Print and shaded views of the part. All mm, measured from the part's lowest x, y and z. A direction names the side the tool comes from. Round coordinates to 2 decimals unless told otherwise and drop trailing zeros. Order: outer loops, then holes, each group sorted by start corner. A loop starts at its lowest first (then second) coordinate and runs counter-clockwise, first axis right, second up. Notation, with made-up numbers: (64, -10) - (85, -10) arc R22 ccw to (85, 28) - close; hole circle Ø9 at (33, 2.5). An arc over 180 degrees is marked (long way). Write item = value, one per line. Start each with the question number.
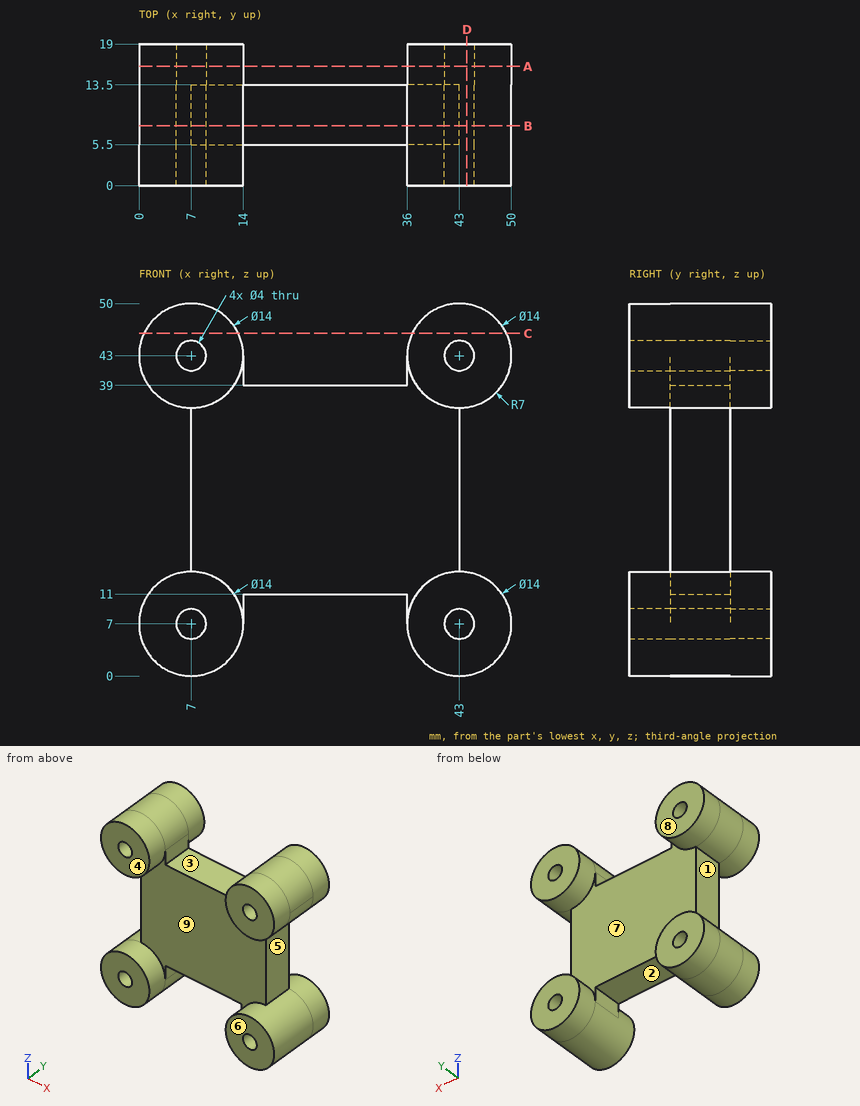
Item 1: Saw through at C-C, the plane z = 46. Give the cut face in (x, y), then the cut area to 3 significant figures.
Item 2: Mould opens along X. For the marked faces 1, 2, 3 and 4 say: +X half, -X half, draft (parallel to the pull), parting line (faces both ways), or undercut.
Item 3: Saw through at B-B, the plane y = 8. Give the cut face in (x, z).
Item 4: Probe L1, parallel to X at y = 17.35, z = 7; L2, parallel to Z at x = 32.5, y = 12.5. List the from-to ranges inside material, lowest first.
Item 5: Saw through at D-D, the plane x = 44. Give the cut face in (y, z).
Item 6: Which spindle directions (+Z, -Z, +X, -X, +Y, -Y) get a long thin tool onto all of the face, cutting with end or side? Do the marked faces 5, 6, 7, 8 and 9. Say none if no direction does.
Item 7: Saw through at A-A, the plane y = 16. Give the cut face in (x, z).
Item 8: Drop flat-ended pins along their axis: pin 1 (6 mm diameter, centred on x = 12.5, y = 4, fed in from +Z); pin 2 (1.2 mm diameter, centred on y = 11.5, z = 41.5, fed in from +X); pin 3 (6.5 mm diameter, centred on x = 25, y = 8.5, fed in from +Z). Give the stop position or say it passes through.
Check sheet entries:
q1.outline = (0.68, 0) - (13.32, 0) - (13.32, 19) - (0.68, 19) - close; (36.68, 0) - (49.32, 0) - (49.32, 19) - (36.68, 19) - close
q1.area = 481 mm2
q2.face_1 = -X half
q2.face_2 = undercut
q2.face_3 = undercut
q2.face_4 = draft
q3.outline = (7, 14) arc R7 ccw (long way) to (14, 7) - (14, 11) - (36, 11) - (36, 7) arc R7 ccw (long way) to (43, 14) - (43, 36) arc R7 ccw (long way) to (36, 43) - (36, 39) - (14, 39) - (14, 43) arc R7 ccw (long way) to (7, 36) - close; hole circle Ø4 at (7, 7); hole circle Ø4 at (7, 43); hole circle Ø4 at (43, 7); hole circle Ø4 at (43, 43)
q4.L1 = 0 to 5, 9 to 14, 36 to 41, 45 to 50
q4.L2 = 11 to 39
q5.outline = (0, 0.07) - (19, 0.07) - (19, 5.27) - (0, 5.27) - close; (0, 8.73) - (19, 8.73) - (19, 13.93) - (0, 13.93) - close; (0, 36.07) - (19, 36.07) - (19, 41.27) - (0, 41.27) - close; (0, 44.73) - (19, 44.73) - (19, 49.93) - (0, 49.93) - close
q6.face_5 = +X, +Y, -Y
q6.face_6 = +Z, -Z, +X, -X, -Y
q6.face_7 = +Y
q6.face_8 = +Z, -Z, +X, -X, +Y
q6.face_9 = -Y
q7.outline = circle Ø14 at (7, 7); circle Ø14 at (7, 43); circle Ø14 at (43, 7); circle Ø14 at (43, 43); hole circle Ø4 at (7, 7); hole circle Ø4 at (7, 43); hole circle Ø4 at (43, 7); hole circle Ø4 at (43, 43)
q8.pin_1 = 49.54
q8.pin_2 = 49.94
q8.pin_3 = 39
